The listing builds one solid part. Answer for the finished solid, in the listing's coordinates (mm). Round coordinates to 2 decimals unless told otherwise and drop trailing zeros. Order: outer loops, then holes, each group sorted by start corner. A loop starts at its lowest first (then second) coordinate and runs counter-clockwise, first axis right, second up. Notation, with made-up numbers: (70.25, 76.5) -> (110.25, 76.5) arc R11 cw to (110.25, 95.5) -> close; hole circle Ø5 at (48, 48). An arc over 180 degrees is marked (long way). Answer in a Markdown table with one row per item. Add a question column.
```python
from build123d import *

# Parameters (mm, degrees)
SKETCH1_R           = 20.25
SKETCH1_R_2         = 2.75
BOSS_EXTRUDE1_DEPTH = 2.8
CHAMFER1_SIZE       = 0.5


with BuildPart() as part:
    # Sketch1 → Boss-Extrude1 (new body)
    with BuildSketch(Plane(origin=(0, 0, 0), x_dir=(1, 0, 0), z_dir=(0, 1, 0))):
        with BuildLine():
            Line((-2.397592731, -65.487125506), (-60.397592731, -65.487125506))
            ThreePointArc((-60.397592731, -65.487125506), (-61.104699513, -65.194232288), (-61.397592731, -64.487125506))
            Line((-61.397592731, -64.487125506), (-61.397592731, -6.487125506))
            ThreePointArc((-61.397592731, -6.487125506), (-61.104699513, -5.780018725), (-60.397592731, -5.487125506))
            Line((-60.397592731, -5.487125506), (-2.397592731, -5.487125506))
            ThreePointArc((-2.397592731, -5.487125506), (-1.69048595, -5.780018725), (-1.397592731, -6.487125506))
            Line((-1.397592731, -6.487125506), (-1.397592731, -64.487125506))
            ThreePointArc((-1.397592731, -64.487125506), (-1.69048595, -65.194232288), (-2.397592731, -65.487125506))
        make_face()
        with Locations((-31.397592731, -35.487125506)):
            Circle(SKETCH1_R, mode=Mode.SUBTRACT)
        with Locations((-54.897592731, -11.987125506)):
            Circle(SKETCH1_R_2, mode=Mode.SUBTRACT)
        with Locations((-7.897592731, -11.987125506)):
            Circle(SKETCH1_R_2, mode=Mode.SUBTRACT)
        with Locations((-7.897592731, -58.987125506)):
            Circle(SKETCH1_R_2, mode=Mode.SUBTRACT)
        with Locations((-54.897592731, -58.987125506)):
            Circle(SKETCH1_R_2, mode=Mode.SUBTRACT)
    extrude(amount=BOSS_EXTRUDE1_DEPTH)

    # Chamfer1
    chamfer1_edges = [part.edges().sort_by_distance(p)[0] for p in [
        (-1.397592731, 0, 35.487125506),
        (-1.69048595, 0, 65.194232288),
        (-31.397592731, 0, 65.487125506),
        (-61.104699513, 0, 65.194232288),
        (-1.69048595, 2.8, 65.194232288),
        (-1.397592731, 2.8, 35.487125506),
        (-1.69048595, 2.8, 5.780018725),
        (-51.647592731, 0, 35.487125506),
        (-51.647592731, 2.8, 35.487125506),
        (-31.397592731, 2.8, 5.487125506),
        (-57.647592731, 0, 11.987125506),
        (-57.647592731, 2.8, 11.987125506),
        (-61.104699513, 2.8, 5.780018725),
        (-10.647592731, 0, 11.987125506),
        (-10.647592731, 2.8, 11.987125506),
        (-61.397592731, 2.8, 35.487125506),
        (-10.647592731, 0, 58.987125506),
        (-10.647592731, 2.8, 58.987125506),
        (-57.647592731, 0, 58.987125506),
        (-57.647592731, 2.8, 58.987125506),
        (-61.104699513, 2.8, 65.194232288),
        (-61.397592731, 0, 35.487125506),
        (-31.397592731, 2.8, 65.487125506),
        (-61.104699513, 0, 5.780018725),
        (-31.397592731, 0, 5.487125506),
        (-1.69048595, 0, 5.780018725),
    ]]
    chamfer(chamfer1_edges, length=CHAMFER1_SIZE)


solid = part.part
```
Item 1: The part is cut by section A-A, the plane y = 1.3. Give the vertices of the cut face in (x, z), and give its area (3 significant figures).
Item 2: For a pull along X with two mould halves and no side action, classify faces 1 (the face through (-61.398, 1, 36)), 2 (the face through (-55.494, 1.387, 61.672)), 3 (the face through (-24, 0, 15)), 4 (the face through (-1.398, 1, 35)) as released by +X, released by -X, zero draft, split by the parting line, or undercut.
Item 3: Find the intervals of material crossed by probe 1 along Z at (x, y) = (-31, 1.3); probe 2 along X at (y, z) = (0.45, 12); probe 3 along X at (y, z) = (0.3, 13), in increasing order. Write a range as [from, to].
Resolved:
| question | item | result |
|---|---|---|
| 1 | outline | (-61.4, 6.49) arc R1 ccw to (-60.4, 5.49) -> (-2.4, 5.49) arc R1 ccw to (-1.4, 6.49) -> (-1.4, 64.49) arc R1 ccw to (-2.4, 65.49) -> (-60.4, 65.49) arc R1 ccw to (-61.4, 64.49) -> close; hole circle Ø5.5 at (-54.9, 11.99); hole circle Ø5.5 at (-54.9, 58.99); hole circle Ø40.5 at (-31.4, 35.49); hole circle Ø5.5 at (-7.9, 11.99); hole circle Ø5.5 at (-7.9, 58.99) |
| 1 | area | 2,220 mm2 |
| 2 | face 1 | released by -X |
| 2 | face 2 | undercut |
| 2 | face 3 | zero draft |
| 2 | face 4 | released by +X |
| 3 | probe 1 | [5.49, 15.24], [55.73, 65.49] |
| 3 | probe 2 | [-61.35, -57.7], [-52.1, -10.7], [-5.1, -1.45] |
| 3 | probe 3 | [-61.2, -57.67], [-52.13, -10.67], [-5.13, -1.6] |
